Source: CAD feature listing. Evaluate the final solid. Frame: model axes, mm. Face numbers are marked on the shaded views. A direction names the side the tool comes from. Round coordinates to 2 decimals unless told otherwise and drop trailing zeros. Write each loop counter-clockwise with the first axis right and the second up, starting at its lowest first coordinate (ties: lowest second). Pieces come first, ordered by that corner, then holes. Notation, with made-up numbers: M 38.25,58 L 52.25,58 A25 cw 52.25,91 Z; hole C -39.75,1.5 d8. An arc over 180 degrees is marked long. Answer in a Markdown table with one row per item. Add a question column.
Item 1: Material intervals for probe 1 along X at (y, z) = (-2.5, 2.15); probe 2 along Y at (x, z) = (-2.5, 0.5); probe 3 along X at (y, z) = (-2.25, 1.7), sorted ascending.
Item 2: Contact query for flat-ended pins moving along their axis: pin 1 (2 mm diameter, centred on x = -1, y = -0.5, fed in from -Z); pin 2 (2 mm diameter, centred on x = 0.5, z = 1.5, fed in from -Y); pin 3 (3 mm diameter, centred on y = 1, z = 1.5, fed in from -X). Output: stop coordinate, or through.
Item 3: Mould query, pull axis X, two halves, no side actions, for the marked faces 1, 2 and 3. Classes: released by +X, released by -X, zero draft, split by the parting line, or undercut.
Item 4: Set-up query: the marked faces 4, 5, 6 and 7. Return all of +Z, -Z, +X, -X, +Y, -Y with unobstructed straight access to the full face (end or side cutting, diameter ignored); none if empty.
Item 5: Cut plane B-B on x = -0.5. Return loops of the section in (y, z).
Item 6: Cut plane C-C on x = 1. Return loops of the section in (y, z).
from build123d import *

# Parameters (mm, degrees)
BOSS_EXTRUDE3_DEPTH = 5


with BuildPart() as part:
    # Sketch1 → Boss-Extrude3 (new body)
    with BuildSketch(Plane.XY):
        with BuildLine():
            Line((3.261099582, 1.194049175), (3.81171563, 1.242385454))
            ThreePointArc((3.81171563, 1.242385454), (3.679113284, 0.539346603), (3.464772438, -0.143225745))
            Line((3.464772438, -0.143225745), (3.997006384, -0.310865928))
            ThreePointArc((3.997006384, -0.310865928), (3.606544346, -0.90817684), (3.148727576, -1.455574989))
            Line((3.148727576, -1.455574989), (3.570884713, -1.8095948))
            ThreePointArc((3.570884713, -1.8095948), (2.981242264, -2.212207675), (2.348432127, -2.542853522))
            Line((2.348432127, -2.542853522), (2.60656535, -3.038366017))
            ThreePointArc((2.60656535, -3.038366017), (1.906611892, -3.184852059), (1.194293663, -3.248063959))
            Line((1.194293663, -3.248063959), (1.242515605, -3.797377559))
            ThreePointArc((1.242515605, -3.797377559), (0.542181479, -3.66545179), (-0.137882302, -3.452412943))
            Line((-0.137882302, -3.452412943), (-0.305258742, -3.983809541))
            ThreePointArc((-0.305258742, -3.983809541), (-0.904553156, -3.591877018), (-1.453561846, -3.132144098))
            Line((-1.453561846, -3.132144098), (-1.809464649, -3.556546643))
            ThreePointArc((-1.809464649, -3.556546643), (-2.211164681, -2.968425537), (-2.541266837, -2.337329731))
            Line((-2.541266837, -2.337329731), (-3.03275883, -2.593368507))
            ThreePointArc((-3.03275883, -2.593368507), (-3.17936368, -1.892614543), (-3.242504481, -1.179478974))
            Line((-3.242504481, -1.179478974), (-3.797247408, -1.228177535))
            ThreePointArc((-3.797247408, -1.228177535), (-3.665254009, -0.527572813), (-3.452085069, 0.152741995))
            Line((-3.452085069, 0.152741995), (-3.978202355, 0.318455585))
            ThreePointArc((-3.978202355, 0.318455585), (-3.587058838, 0.916685937), (-3.128354184, 1.464830849))
            Line((-3.128354184, 1.464830849), (-3.556416492, 1.823802719))
            ThreePointArc((-3.556416492, 1.823802719), (-2.966435761, 2.226618489), (-2.333244393, 2.55738502))
            Line((-2.333244393, 2.55738502), (-2.587761321, 3.045955674))
            ThreePointArc((-2.587761321, 3.045955674), (-1.889660833, 3.19216629), (-1.179234612, 3.255541529))
            Line((-1.179234612, 3.255541529), (-1.228047384, 3.811585479))
            ThreePointArc((-1.228047384, 3.811585479), (-0.524737953, 3.678915376), (0.158085284, 3.464444075))
            Line((0.158085284, 3.464444075), (0.324062771, 3.991399198))
            ThreePointArc((0.324062771, 3.991399198), (0.92030935, 3.601725697), (1.466842606, 3.144936008))
            Line((1.466842606, 3.144936008), (1.82393287, 3.570754562))
            ThreePointArc((1.82393287, 3.570754562), (2.227660979, 2.979252099), (2.558969454, 2.344345616))
            Line((2.558969454, 2.344345616), (3.05156286, 2.600958164))
            ThreePointArc((3.05156286, 2.600958164), (3.197654322, 1.903658089), (3.261099582, 1.194049175))
        make_face()
    extrude(amount=BOSS_EXTRUDE3_DEPTH)


solid = part.part
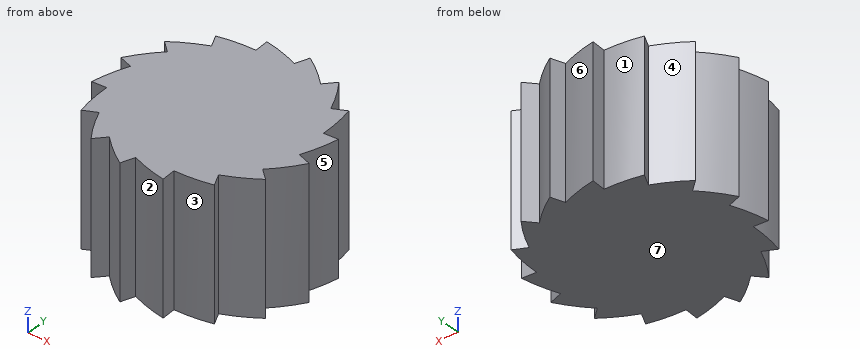
Results below:
| question | item | result |
|---|---|---|
| 1 | probe 1 | -3.06 to -2.85, -2.47 to 2.44 |
| 1 | probe 2 | -2.43 to 2.48, 2.88 to 3.07 |
| 1 | probe 3 | -3.12 to 2.92 |
| 2 | pin 1 | z = 0 |
| 2 | pin 2 | y = -3.98 |
| 2 | pin 3 | x = -3.98 |
| 3 | face 1 | released by -X |
| 3 | face 2 | undercut |
| 3 | face 3 | released by +X |
| 4 | face 4 | +Z, -Z, -X |
| 4 | face 5 | +Z, -Z, +X |
| 4 | face 6 | +Z, -Z, +Y |
| 4 | face 7 | -Z, +X, -X, +Y, -Y |
| 5 | outline | M -3.87,0 L 3.67,0 L 3.67,5 L -3.87,5 Z |
| 6 | outline | M -3.76,0 L 3.54,0 L 3.54,5 L -3.76,5 Z |
